Geometry: see drawing. Coordinates: mm, zero at the bounding-box minimum. A direction names the side the tool comes from. Give positions to 0.01 mm unless a question says otherwise; leave off trailing zeros. Order: outer loops, then holes, each group sorted by start corner. A loop starts at its lowest first (then second) coordinate and runs counter-clockwise, first axis right, second up. Notation, with made-up numbers: M -10,45.5 L 49,45.5 A8 cw 49,60.5 Z; hole C 52.5,-11.5 d11. An arc over 180 degrees is marked long. Write item = value, one per line. Start each with the question number.
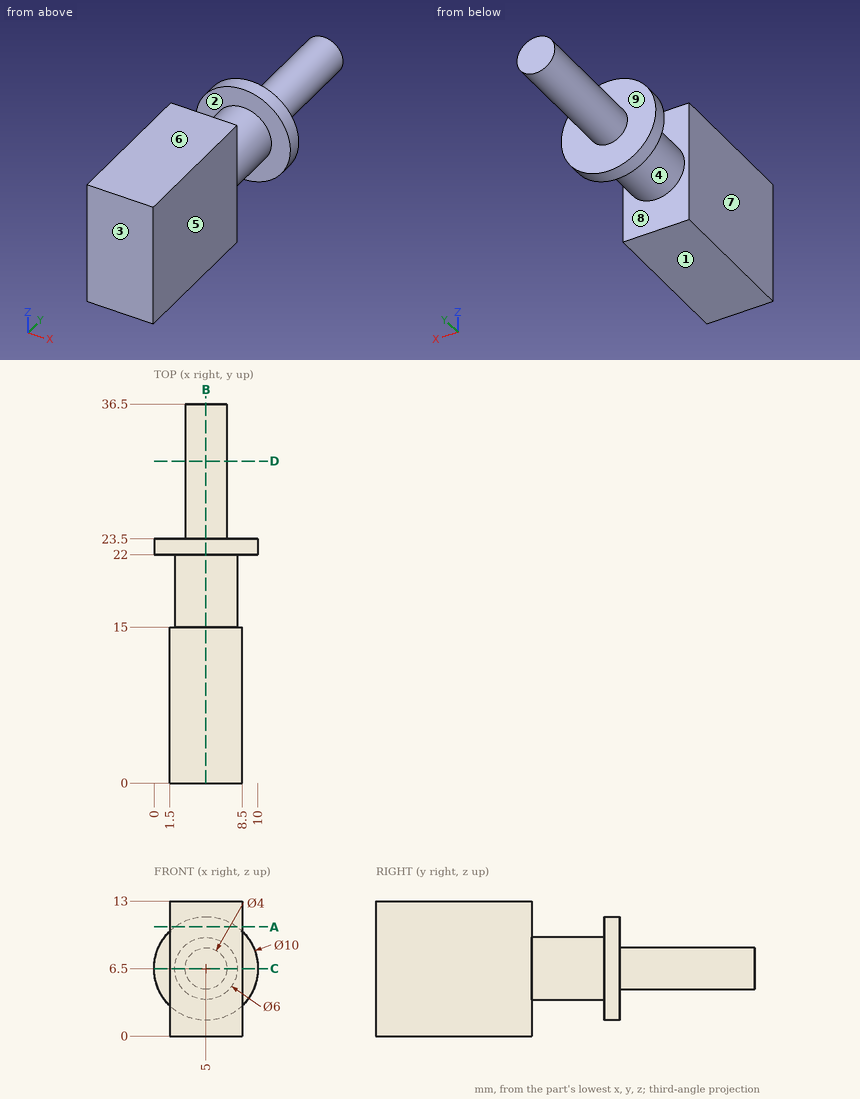
1) Draft query along Y for the marked faces 1, 2, 3 and 4. Return one class per face: pulls with the +Y half, pulls with the -Y half, needs draft (parallel to the pull), parting line crosses it, or undercut.
2) Cut plane B-B (x = 5). Return loops of the section in (y, z).
3) Ray query, L1, parallel to Y at x = 6, z = 11; L2, parallel to X at y = 2, z = 12; L3, parallel to Y at x = 7.5, z = 2. Return the intervals inside material, ascending.
4) Cut plane D-D (y = 31). Return loops of the section in (x, z).
5) Cut plane A-A (z = 10.5). Return loops of the section in (x, y), plus the area to 3 significant figures.
6) Cut plane C-C (z = 6.5). Return loops of the section in (x, y), plus the area to 3 significant figures.
7) Pin query (flat end, axial travel): pin 1 Ø5 at (y, z) = (7.5, 2) entering from +X; pin 2 Ø4 at (x, y) = (7.5, 29) entering from -Z; pin 3 Ø3 at (x, y) = (5.5, 22.5) entering from +Z. Return the tip coordinate at first contact, or that it passes through.
8) Access query for the marked faces 5, 6, 7, 8 and 9. Directions: +Z, -Z, +X, -X, +Y, -Y. A direction counts if a zero-diameter tool reaches every point of the face in a straight line with its end or side. Return the directions, or none.
Reply:
q1.face_1 = needs draft
q1.face_2 = undercut
q1.face_3 = pulls with the -Y half
q1.face_4 = undercut
q2.outline = M 0,0 L 15,0 L 15,3.5 L 22,3.5 L 22,1.5 L 23.5,1.5 L 23.5,4.5 L 36.5,4.5 L 36.5,8.5 L 23.5,8.5 L 23.5,11.5 L 22,11.5 L 22,9.5 L 15,9.5 L 15,13 L 0,13 Z
q3.L1 = 0 to 15, 22 to 23.5
q3.L2 = 1.5 to 8.5
q3.L3 = 0 to 15
q4.outline = C 5,6.5 d4
q5.outline = M 1.5,0 L 8.5,0 L 8.5,15 L 1.5,15 Z; M 2,22 L 8,22 L 8,23.5 L 2,23.5 Z
q5.area = 114 mm²
q6.outline = M 0,22 L 2,22 L 2,15 L 1.5,15 L 1.5,0 L 8.5,0 L 8.5,15 L 8,15 L 8,22 L 10,22 L 10,23.5 L 7,23.5 L 7,36.5 L 3,36.5 L 3,23.5 L 0,23.5 Z
q6.area = 214 mm²
q7.pin_1 = 8.5
q7.pin_2 = 4.56
q7.pin_3 = 11.5
q8.face_5 = +Z, -Z, +X, -Y
q8.face_6 = +Z, +X, -X, +Y, -Y
q8.face_7 = +Z, -Z, -X, -Y
q8.face_8 = none
q8.face_9 = +Y
